Geometry: see drawing. Coordinates: mm, zero at the bounding-box minimum. A direction names the side the tool comes from. Coordinates: 2 decimals unless noted, no trailing zeros. Write each loop counter-clockwise with the first axis right and the second up, starting at its lowest first coordinate (ties: lowest second). Pieces come first, ordered by that corner, then holes. Notation, with made-up numbers: (6.5, -32.5) - (24.5, -32.5) arc R31 ccw to (24.5, -1.5) - close; hole circle Ø4 at (51, 22). An arc over 180 degrees is marked (long way). Use a Markdown table: item, result. Add a question column.
Q1. Section query C-C (x = 13.5). Return the cut outline in (y, z), then the cut area to 3 significant figures.
Q2. Pin query (flat end, axial travel): P1, Ø4, axis at y = 26, z = 6.5, coming from the +X side; P2, Ø1, axis at y = 4.5, z = 4, coming from the -X side; P3, Ø0.8, axis at x = 4, z = 5.5, coming from the -Y side. Return the tip coordinate at first contact, or that it passes through.
Q3. Material intervals for probe 1 along Y at (x, z) = (19, 5.5); probe 2 along X at (y, z) = (20, 7); probe 3 along Y at (x, z) = (19, 7.5), sorted ascending. Write a range as from..to.
Q4. Section query A-A (x = 3). Return the cut outline in (y, z) (1 decimal).
Q5. Set-up query: the marked faces 1, 2, 3, 4 and 5. Return all of +Z, -Z, +X, -X, +Y, -Y with unobstructed straight access to the full face (end or side cutting, diameter ignored); none if empty.
Q6. Section query D-D (y = 3.25). Return the cut outline in (x, z).
Q7. Mould query, pull axis Y, two halves, no side actions, for the marked faces 6, 7 and 8. Classes: released by +Y, released by -Y, zero draft, split by the parting line, or undercut.
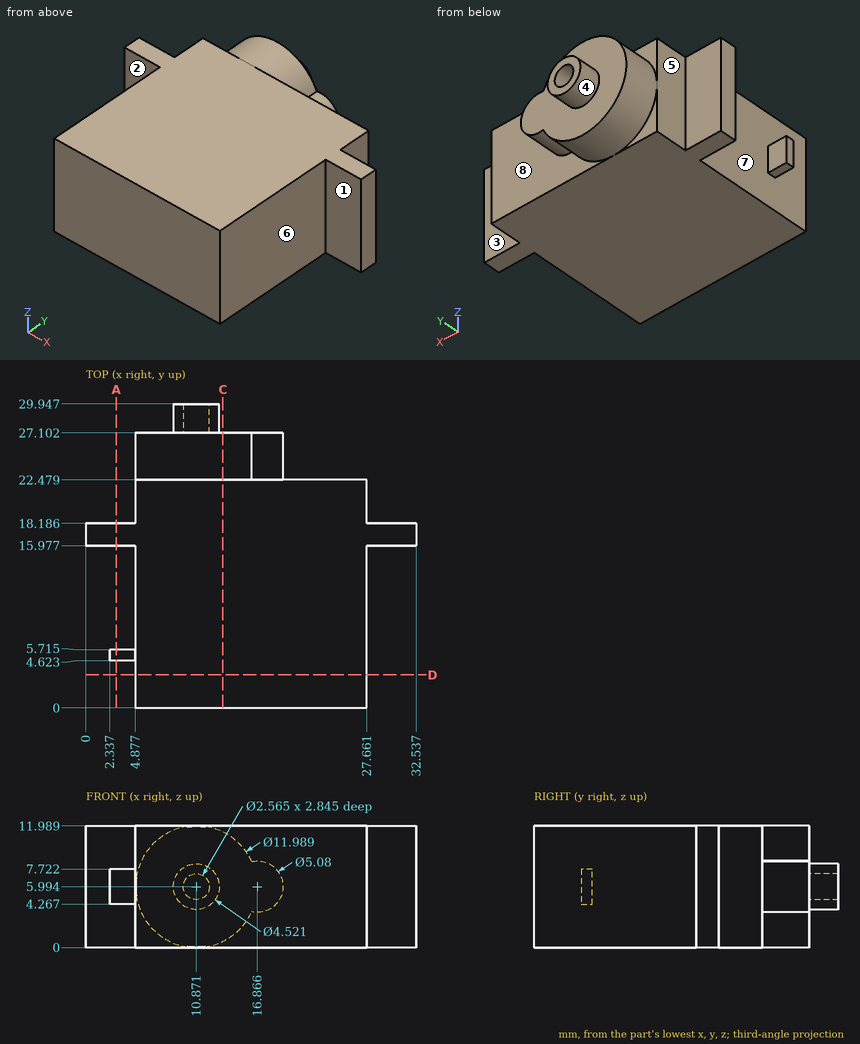
Values follow:
| question | item | result |
|---|---|---|
| 1 | outline | (0, 0) - (22.48, 0) - (22.48, 0.61) - (27.1, 0.61) - (27.1, 11.38) - (22.48, 11.38) - (22.48, 11.99) - (0, 11.99) - close |
| 1 | area | 319 mm2 |
| 2 | P1 | x = 19.41 |
| 2 | P2 | x = 2.34 |
| 2 | P3 | y = 4.62 |
| 3 | probe 1 | 0..27.1 |
| 3 | probe 2 | 4.88..27.66 |
| 3 | probe 3 | 0..22.48 |
| 4 | outline | (4.6, 4.3) - (5.7, 4.3) - (5.7, 7.7) - (4.6, 7.7) - close; (16, 0) - (18.2, 0) - (18.2, 12) - (16, 12) - close |
| 5 | face 1 | +Z, -Z, +X, -Y |
| 5 | face 2 | +Z, -Z, -X |
| 5 | face 3 | +Z, -Z, +X, +Y |
| 5 | face 4 | +Y |
| 5 | face 5 | +Z, -Z, -X, +Y |
| 6 | outline | (4.88, 0) - (27.66, 0) - (27.66, 11.99) - (4.88, 11.99) - close |
| 7 | face 6 | zero draft |
| 7 | face 7 | undercut |
| 7 | face 8 | released by +Y |
